Design review of the part built by this model. Coordinates are the model's own, in mm. Coordinates: 2 decimals unless noted, no trailing zeros. Write item = value, one per line.
```python
from build123d import *

# Parameters (mm, degrees)
SKETCH1_W           = 210
SKETCH1_H           = 450
SKETCH1_W_2         = 150
SKETCH1_H_2         = 15
BOSS_EXTRUDE1_DEPTH = 3
SKETCH3_W           = 3
SKETCH3_H           = 24
BOSS_EXTRUDE3_DEPTH = 3
SKETCH2_W           = 24
SKETCH2_H           = 3
BOSS_EXTRUDE4_DEPTH = 3


with BuildPart() as part:
    # Sketch1 → Boss-Extrude1 (new body)
    with BuildSketch(Plane(origin=(0, 0, 0), x_dir=(1, 0, 0), z_dir=(0, 1, 0))):
        Rectangle(SKETCH1_W, SKETCH1_H)
        with Locations((0, -162.5)):
            Rectangle(SKETCH1_W_2, SKETCH1_H_2, mode=Mode.SUBTRACT)
        with Locations((0, -187.5)):
            Rectangle(SKETCH1_W_2, SKETCH1_H_2, mode=Mode.SUBTRACT)
        with Locations((0, -137.5)):
            Rectangle(SKETCH1_W_2, SKETCH1_H_2, mode=Mode.SUBTRACT)
        with Locations((0, -112.5)):
            Rectangle(SKETCH1_W_2, SKETCH1_H_2, mode=Mode.SUBTRACT)
        with Locations((0, -87.5)):
            Rectangle(SKETCH1_W_2, SKETCH1_H_2, mode=Mode.SUBTRACT)
        with Locations((0, -62.5)):
            Rectangle(SKETCH1_W_2, SKETCH1_H_2, mode=Mode.SUBTRACT)
        with Locations((0, -37.5)):
            Rectangle(SKETCH1_W_2, SKETCH1_H_2, mode=Mode.SUBTRACT)
        with Locations((0, -12.5)):
            Rectangle(SKETCH1_W_2, SKETCH1_H_2, mode=Mode.SUBTRACT)
        with Locations((0, 12.5)):
            Rectangle(SKETCH1_W_2, SKETCH1_H_2, mode=Mode.SUBTRACT)
        with Locations((0, 37.5)):
            Rectangle(SKETCH1_W_2, SKETCH1_H_2, mode=Mode.SUBTRACT)
        with Locations((0, 62.5)):
            Rectangle(SKETCH1_W_2, SKETCH1_H_2, mode=Mode.SUBTRACT)
        with Locations((0, 87.5)):
            Rectangle(SKETCH1_W_2, SKETCH1_H_2, mode=Mode.SUBTRACT)
        with Locations((0, 112.5)):
            Rectangle(SKETCH1_W_2, SKETCH1_H_2, mode=Mode.SUBTRACT)
        with Locations((0, 137.5)):
            Rectangle(SKETCH1_W_2, SKETCH1_H_2, mode=Mode.SUBTRACT)
        with Locations((0, 162.5)):
            Rectangle(SKETCH1_W_2, SKETCH1_H_2, mode=Mode.SUBTRACT)
        with Locations((0, 187.5)):
            Rectangle(SKETCH1_W_2, SKETCH1_H_2, mode=Mode.SUBTRACT)
    extrude(amount=BOSS_EXTRUDE1_DEPTH)

    # Sketch3 → Boss-Extrude3 (add)
    with BuildSketch(Plane(origin=(0, 3, 0), x_dir=(1, 0, 0), z_dir=(0, 1, 0))):
        with Locations((-106.5, 192)):
            Rectangle(SKETCH3_W, SKETCH3_H)
        with Locations((106.5, 192)):
            Rectangle(SKETCH3_W, SKETCH3_H)
        with Locations((106.5, 144)):
            Rectangle(SKETCH3_W, SKETCH3_H)
        with Locations((106.5, 96)):
            Rectangle(SKETCH3_W, SKETCH3_H)
        with Locations((106.5, 48)):
            Rectangle(SKETCH3_W, SKETCH3_H)
        with Locations((106.5, 0)):
            Rectangle(SKETCH3_W, SKETCH3_H)
        with Locations((106.5, -48)):
            Rectangle(SKETCH3_W, SKETCH3_H)
        with Locations((106.5, -96)):
            Rectangle(SKETCH3_W, SKETCH3_H)
        with Locations((106.5, -144)):
            Rectangle(SKETCH3_W, SKETCH3_H)
        with Locations((106.5, -192)):
            Rectangle(SKETCH3_W, SKETCH3_H)
        with Locations((-106.5, 144)):
            Rectangle(SKETCH3_W, SKETCH3_H)
        with Locations((-106.5, 96)):
            Rectangle(SKETCH3_W, SKETCH3_H)
        with Locations((-106.5, 48)):
            Rectangle(SKETCH3_W, SKETCH3_H)
        with Locations((-106.5, 0)):
            Rectangle(SKETCH3_W, SKETCH3_H)
        with Locations((-106.5, -48)):
            Rectangle(SKETCH3_W, SKETCH3_H)
        with Locations((-106.5, -96)):
            Rectangle(SKETCH3_W, SKETCH3_H)
        with Locations((-106.5, -144)):
            Rectangle(SKETCH3_W, SKETCH3_H)
        with Locations((-106.5, -192)):
            Rectangle(SKETCH3_W, SKETCH3_H)
    extrude(amount=-BOSS_EXTRUDE3_DEPTH)

    # Sketch2 → Boss-Extrude4 (add)
    with BuildSketch(Plane(origin=(0, 3, 0), x_dir=(1, 0, 0), z_dir=(0, 1, 0))):
        with Locations((-72, 226.5)):
            Rectangle(SKETCH2_W, SKETCH2_H)
        with Locations((-24, 226.5)):
            Rectangle(SKETCH2_W, SKETCH2_H)
        with Locations((24, 226.5)):
            Rectangle(SKETCH2_W, SKETCH2_H)
        with Locations((72, 226.5)):
            Rectangle(SKETCH2_W, SKETCH2_H)
        with Locations((-71.999992971, -226.5)):
            Rectangle(SKETCH2_W, SKETCH2_H)
        with Locations((-23.999992971, -226.5)):
            Rectangle(SKETCH2_W, SKETCH2_H)
        with Locations((24.000007029, -226.5)):
            Rectangle(SKETCH2_W, SKETCH2_H)
        with Locations((72.000007029, -226.5)):
            Rectangle(SKETCH2_W, SKETCH2_H)
    extrude(amount=-BOSS_EXTRUDE4_DEPTH)


solid = part.part
```
Q1. Wall thickness on line 1 (X direction, y = 2.45, z = -16.5); line 2 (Z direction, x = -89, y = 1.3); line 3 (X direction, y = 0.7, z = -106): over which ranges is each line inside the solid? List them lowest first.
Check result:
line_1 = -105 to -75, 75 to 105
line_2 = -225 to 225
line_3 = -108 to -75, 75 to 108
Q2. For P1, Ø1.5, axis at y = 1, z = -226, coming from the +X side; P2, Ø1.5, axis at x = 106.5, y = 1.5, coming from the +Z side; P3, Ø1.5, axis at x = 51.5, y = 1.5, coming from the -Z side; P4, Ø2, axis at x = -37, z = -144.5, coming from the +Y side, all flat-tipped, find the tip position at first contact; note any pin that passes through.
Check result:
P1 = 84
P2 = 204
P3 = -225
P4 = 3
Q3. Consider section A-A, the plane x = -5.5. State how many separate pieces and enclosed holes the cut face has, and give its area (3 significant figures).
Check result:
separate_pieces = 17
enclosed_holes = 0
area = 630 mm²
